Autodesk Inventor part; units mm, degrees
ref_plane "YZ Plane" through (0, 0, 0) normal (1, 0, 0) x (0, 1, 0)
ref_plane "XZ Plane" through (0, 0, 0) normal (0, 1, 0) x (-1, 0, 0)
ref_plane "XY Plane" through (0, 0, 0) normal (0, 0, 1) x (1, 0, 0)
ref_plane "Arbeitsebene1" through (-0.0002, 0, 0) normal (0, 0, 1) x (1, 0, 0)
sketch "Skizze1" plane through (-0.0002, 0, 0) normal (0, 0, 1) x (1, 0, 0)
  circle A0 centre (13.85, 6.86) radius 1.5
  circle A1 centre (0.85, 31.86) radius 1.5
  circle A2 centre (13.85, 31.86) radius 1.5
  circle A3 centre (0.85, 6.86) radius 1.5
  circle A4 centre (5.0933, 19.36) radius 5.5
  line L0 (-3.07, 5.49) -> (-3.07, 33.23)
  line L1 (-3.07, 5.49) -> (-16.87, 5.49)
  line L2 (-16.87, 13.31) -> (-16.87, 5.49)
  line L3 (-16.8476, 13.31) -> (-16.87, 13.31)
  line L4 (-16.8476, 25.41) -> (-16.8476, 13.31)
  line L5 (-16.87, 25.41) -> (-16.8476, 25.41)
  line L6 (-16.87, 33.23) -> (-16.87, 25.41)
  line L7 (-3.07, 33.23) -> (-16.87, 33.23)
  line L8 (-16.87, 40.13) -> (-16.87, 44.21)
  line L9 (-20.77, 36.23) -> (-16.87, 40.13)
  line L10 (-24.85, 36.23) -> (-20.77, 36.23)
  line L11 (-24.85, 2.49) -> (-24.85, 36.23)
  line L12 (-20.77, 2.49) -> (-24.85, 2.49)
  line L13 (-16.87, -1.41) -> (-20.77, 2.49)
  line L14 (-16.87, -1.41) -> (-16.87, -5.49)
  line L15 (-16.87, -5.49) -> (16.87, -5.49)
  line L16 (16.87, -5.49) -> (16.87, -1.41)
  line L17 (20.77, 2.49) -> (16.87, -1.41)
  line L18 (24.85, 2.49) -> (20.77, 2.49)
  line L19 (24.85, 36.23) -> (24.85, 2.49)
  line L20 (20.77, 36.23) -> (24.85, 36.23)
  line L21 (16.87, 40.13) -> (20.77, 36.23)
  line L22 (16.87, 44.21) -> (16.87, 40.13)
  line L23 (-16.87, 44.21) -> (16.87, 44.21)
  line L24 (16.97, 36.33) -> (16.97, 2.39)
  line L25 (-16.97, 36.33) -> (16.97, 36.33) construction
  line L26 (-16.97, 2.39) -> (-16.97, 36.33)
  line L27 (16.97, 2.39) -> (-16.97, 2.39) construction
  line L28 (16.97, 2.39) -> (-16.97, 2.39)
  line L29 (16.47, 35.83) -> (16.47, 2.89)
  line L30 (16.47, 2.89) -> (-16.47, 2.89)
  line L31 (-16.47, 2.89) -> (-16.47, 35.83)
  line L32 (-16.47, 35.83) -> (16.47, 35.83)
  line L33 (-2.57, 35.83) -> (-2.57, 2.89)
  circle A5 centre (5.0933, 19.36) radius 7
  point P0 (0.0002, 0)
  dimension "d0" = 0.5
  dimension "d1" = 0.5
  dimension "d18" = 14
extrude "Extrusion1" add sketch "Skizze1" along normal blind 25 contours L33 L32 L29 L30
sketch "Skizze2" plane through (-2.5702, 2.89, 0) normal (0, -1, 0) x (1, 0, 0)
  line L0 (0, 0) -> (0, 25)
  line L1 (0, 25) -> (-3, 25)
  line L2 (-3, 25) -> (-3, 15)
  line L3 (-3, 15) -> (0, 15)
  line L4 (0, 15) -> (0, 25)
  point P0 (2.5702, 0)
  point P1 (0, 15)
  dimension "d4" = 3
  dimension "d5" = 10
extrude "Extrusion2" add sketch "Skizze2" against normal up to surface (32.94 mm away)
sketch "Skizze3" plane through (-0.0002, 0, 0) normal (0, 0, -1) x (-1, 0, 0)
  circle A0 centre (2.4634, 11.66) radius 1
  circle A1 centre (-13.85, 6.86) radius 1.5
  circle A2 centre (-12.9366, 27.06) radius 1
  circle A3 centre (2.4634, 27.06) radius 1
  circle A4 centre (-12.9366, 27.06) radius 1
  arc A5 (-14.6686, 11.41) -> (-13.1866, 9.9279) centre (-12.9366, 11.66) ccw
  arc A6 (-13.1866, 13.3921) -> (-14.6686, 11.91) centre (-12.9366, 11.66) ccw
  point P0 (-0.0002, 0)
hole "Bohrung1" at (-2.4636, 11.66, 0) at (-2.4636, 27.06, 0) at (12.9364, 27.06, 0) at (12.9364, 11.66, 0) direction (0, 0, 1) diameter 2.5 end through all counterbore diameter 5 counterbore depth 18
sketch "Skizze4" plane through (-0.0002, 0, 25) normal (0, 0, 1) x (1, 0, 0)
  circle A0 centre (5.0933, 19.36) radius 5.5
  circle A1 centre (5.0933, 19.36) radius 9.5
  point P0 (0.0002, 0)
  dimension "d15" = 19
extrude "Extrusion3" cut sketch "Skizze4" against normal blind 4 contours A0 | A1
properties part number "30_Cube_Z_Focus_NEMA8_captive_motorbase_v0"
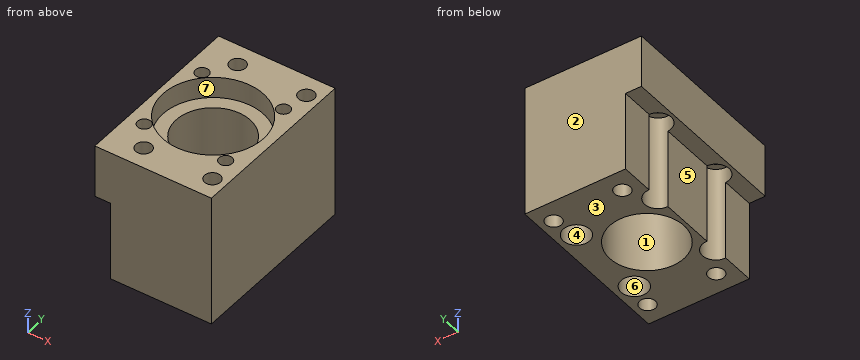
Input: part model. Units: mm. Frame: model coordinates. Face numbers are marked on the shaded views. A direction names the side the tool comes from. Coordinates: 2 decimals unless noted, no trailing zeros. Loops run counter-clockwise (first coordinate to the right, second up) from the corner with the lowest first, then second, coordinate; pieces in that order, holes last. Notation, with made-up numbers: (68, 28.25) -> (92, 28.25) arc R28 cw to (92, 47.25) -> close; hole circle Ø10 at (72.25, 68). An arc over 180 degrees is marked (long way). Use a Markdown table: item, result.
1) Material intervals for line 1 along X through (y, z) = (32, 12); line 2 along Y through (x, z) = (-2, 4.75); line 3 along Y through (x, z) = (5.5, 21.5), sorted ascending. Write a range as from..to.
Results found:
| item | result |
|---|---|
| line 1 | x = -2.57..-0.64, 2.34..12.36, 15.34..16.47 |
| line 2 | y = 2.89..9.2, 14.12..24.6, 29.52..35.83 |
| line 3 | y = 2.89..9.87, 28.85..35.83 |
2) Pull-direction query (Y, two-part tool) for the marked faces 1, 2, 3 and 4; classes: released by +Y, released by -Y, zero draft, split by the parting line, or undercut.
Results found:
| item | result |
|---|---|
| face 1 | undercut |
| face 2 | released by +Y |
| face 3 | zero draft |
| face 4 | undercut |
3) Contact query for flat-ended pins moving along their axis: pin 1 (4 mm diameter, centred on x = -2.5, y = 11, fed in from -Z); pin 2 (5 mm diameter, centred on y = 31, z = 10, fed in from -X); pin 3 (1.5 mm diameter, centred on x = 12.94, y = 11.66, fed in from -Z); pin 4 (4 mm diameter, centred on x = 12.94, y = 27.06, fed in from -Z). Output: stop coordinate, or through.
Results found:
| item | result |
|---|---|
| pin 1 | stops at z = 0 |
| pin 2 | stops at x = -2.57 |
| pin 3 | passes through |
| pin 4 | stops at z = 18 |
4) Cut plane D-D (z = 8). Return the cut outline in (x, y), then the cut area to 3 significant figures.
Results found:
| item | result |
|---|---|
| outline | (-2.57, 2.89) -> (16.47, 2.89) -> (16.47, 35.83) -> (-2.57, 35.83) -> (-2.57, 29.56) arc R2.5 cw (long way) to (-2.57, 24.56) -> (-2.57, 14.16) arc R2.5 cw (long way) to (-2.57, 9.16) -> close; hole circle Ø14 at (5.09, 19.36); hole circle Ø3 at (0.85, 6.86); hole circle Ø3 at (0.85, 31.86); hole circle Ø5 at (12.94, 11.66); hole circle Ø5 at (12.94, 27.06); hole circle Ø3 at (13.85, 6.86); hole circle Ø3 at (13.85, 31.86) |
| area | 385 mm2 |
5) Cut plane C-C (x = -3). Return the cut outline in (y, z), then the cut area to 3 significant figures.
Results found:
| item | result |
|---|---|
| outline | (2.89, 15) -> (9.22, 15) -> (9.22, 18) -> (10.53, 18) -> (10.53, 25) -> (2.89, 25) -> close; (12.79, 18) -> (14.1, 18) -> (14.1, 15) -> (24.62, 15) -> (24.62, 18) -> (25.93, 18) -> (25.93, 25) -> (24.34, 25) -> (24.34, 21) -> (14.38, 21) -> (14.38, 25) -> (12.79, 25) -> close; (28.19, 18) -> (29.5, 18) -> (29.5, 15) -> (35.83, 15) -> (35.83, 25) -> (28.19, 25) -> close |
| area | 229 mm2 |
6) Cut plane A-A (y = 19.36). Return the cut outline in (x, z).
Results found:
| item | result |
|---|---|
| outline | (-5.57, 15) -> (-2.57, 15) -> (-2.57, 0) -> (-1.91, 0) -> (-1.91, 21) -> (-4.41, 21) -> (-4.41, 25) -> (-5.57, 25) -> close; (12.09, 0) -> (16.47, 0) -> (16.47, 25) -> (14.59, 25) -> (14.59, 21) -> (12.09, 21) -> close |
7) Access query for the marked faces 5, 6 and 7. Directions: +Z, -Z, +X, -X, +Y, -Y. A direction counts if a zero-diameter tool reaches every point of the face in a straight line with its end or side. Return the directions, or none.
Results found:
| item | result |
|---|---|
| face 5 | -Z, -X, +Y, -Y |
| face 6 | -Z |
| face 7 | +Z |
8) Cut plane B-B (y = 6.86). Return the cut outline in (x, z), then the cut area to 3 significant figures.
Results found:
| item | result |
|---|---|
| outline | (-5.57, 15) -> (-2.57, 15) -> (-2.57, 0) -> (-0.65, 0) -> (-0.65, 25) -> (-5.57, 25) -> close; (2.35, 0) -> (12.35, 0) -> (12.35, 25) -> (2.35, 25) -> close; (15.35, 0) -> (16.47, 0) -> (16.47, 25) -> (15.35, 25) -> close |
| area | 356 mm2 |
